Build history of the part. All positions in model axes, mm. Face numbers are marked on the shaded views. A direction names the side the tool comes from. Round coordinates to 2 decimals unless told otherwise and drop trailing zeros. Write each loop counter-clockwise with the first axis right and the second up, starting at its lowest first coordinate (ties: lowest second). Pieces come first, ordered by that corner, then holes. Notation, with made-up numbers: (78.25, -31.75) -> (127.25, -31.75) arc R16 cw to (127.25, -22.75) -> close; hole circle Ø4 at (24, 63.5). An arc over 180 degrees is marked (long way). Return JSON: item names as keys, results as strings.
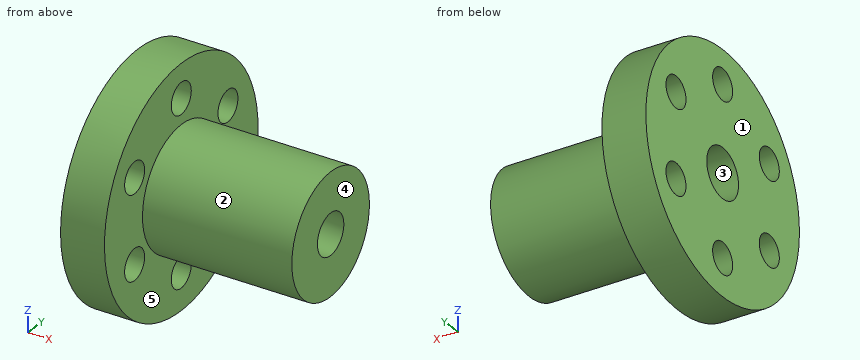
from build123d import *

# Parameters (mm, degrees)
F2_R     = 2.130745
F3_DEPTH = 6.001


with BuildPart() as f1:
    # F0 (on Front) → F1 (revolve)
    with BuildSketch(Plane.XZ):
        Polygon((-5.551115, 16.115252), (-11.551115, 16.115252), (-11.551115, 3.144817), (14.848885, 2.570904), (14.848885, 8.023078), (-5.551115, 8.023078), align=None)
    revolve(axis=Axis((0.128016, 0, -0.24127), (1, 0, 0)))

    # F2 (on face) → F3 (cut, through all)
    with BuildSketch(Plane.YZ.offset(-5.551115)):
        with Locations((-9.941192, 5.73955)):
            Circle(F2_R)
        with Locations((-9.941192, -5.73955)):
            Circle(F2_R)
        with Locations((0, -11.479099)):
            Circle(F2_R)
        with Locations((9.941192, -5.73955)):
            Circle(F2_R)
        with Locations((9.941192, 5.73955)):
            Circle(F2_R)
        with Locations((0, 11.479099)):
            Circle(F2_R)
    extrude(amount=-F3_DEPTH, mode=Mode.SUBTRACT)


solid = f1.part
Q1. 3-axis set-ups, long thin cutter, end or side, ignore diameter. For the marked faces 4 and 5: which of +Z, -Z, +X, -X, +Y, -Y reach the whole face in a straight line?
Verdict:
{"face 4": "+Z, -Z, +X, +Y, -Y", "face 5": "+X"}
Q2. Saw through at C-C on x = -7.75. List the corners of the cut face in (y, z), then the cut area to 3 significant figures.
Verdict:
{"outline": "circle Ø32.71 at (0, -0.24); hole circle Ø4.26 at (-9.94, -5.74); hole circle Ø4.26 at (-9.94, 5.74); hole circle Ø6.61 at (0, -0.24); hole circle Ø4.26 at (0, -11.48); hole circle Ø4.26 at (0, 11.48); hole circle Ø4.26 at (9.94, -5.74); hole circle Ø4.26 at (9.94, 5.74)", "area": "721 mm²"}
Q3. Saw through at A-A on z = -12. List the corners of the cut face in (x, y).
Verdict:
{"outline": "(-11.55, -11.37) -> (-5.55, -11.37) -> (-5.55, -2.07) -> (-11.55, -2.07) -> close; (-11.55, 2.07) -> (-5.55, 2.07) -> (-5.55, 11.37) -> (-11.55, 11.37) -> close"}
Q4. Two-plate mould, pull along Y, no slides. Class the marked faces 1, 2 and 3: +Y half, -Y half, draft (parallel to the pull), parting line (faces both ways), or undercut.
Verdict:
{"face 1": "draft", "face 2": "parting line", "face 3": "undercut"}
Q5. Pin check, flat tips, straight feed: pin 1 Ø2.5 at (y, z) = (-9.94, -5.74) entering from -X; pin 2 Ø1.5 at (x, z) = (-1.5, -8.5) entering from -Y; pin 3 Ø8 at (x, y) = (0.5, 3) entering from -Z; pin 4 Ø6 at (x, y) = (11.5, 4) entering from +Z. Stop position of each tip, or through.
Verdict:
{"pin 1": "passes through", "pin 2": "stops at y = -3.45", "pin 3": "stops at z = -8.51", "pin 4": "stops at z = 7.96"}
Q6. Wall check: L1, parallel to X at y = -3, z = -13; L2, parallel to Z at x = -7.65, y = 0; L3, parallel to Z at x = -4.5, y = -0.5. Give the ranges that are in metal, low to high.
Verdict:
{"L1": "x = -11.55 to -5.55", "L2": "z = -16.6 to -13.61, -9.35 to -3.54, 3.06 to 9.35, 13.61 to 16.12", "L3": "z = -8.49 to -3.44, 2.95 to 8.01"}
Q7. Saw through at B-B on z = 5. List the corners of the cut face in (x, y).
Verdict:
{"outline": "(-11.55, -15.49) -> (-5.55, -15.49) -> (-5.55, -11.94) -> (-11.55, -11.94) -> close; (-11.55, -7.94) -> (-5.55, -7.94) -> (-5.55, -6.39) -> (14.85, -6.39) -> (14.85, 6.39) -> (-5.55, 6.39) -> (-5.55, 7.94) -> (-11.55, 7.94) -> close; (-11.55, 11.94) -> (-5.55, 11.94) -> (-5.55, 15.49) -> (-11.55, 15.49) -> close"}
Q8. Saw through at D-D on y = -1. Count the separate pieces of the cut face and the enclosed holes in it, then the cut area to 3 significant figures.
Verdict:
{"separate pieces": "4", "enclosed holes": "0", "area": "331 mm²"}
